Input: dimensioned drawing with shaded views. Units: mm. Origin: part minimum x, y, z. A direction names the side the tool comes from. Round coordinates to 2 decimals unless told otherwise and drop trailing zeros. Loops run counter-clockwise (first coordinate to the right, second up) from the corner with the lowest first, then second, coordinate; pieces in that order, holes last.
Item 1: Section query A-A on z = 16.5. Return loops of the section in (x, y), then the cut area to 3 significant figures.
Item 2: First-contact query: P1, Ø1.5, axis at y = 2.5, z = 10.5, coming from the +X side; P2, Ø2.5, axis at x = 6, z = 16.5, coming from the +Y side; P3, Ø0.9, axis at x = 6, z = 6.5, coming from the -Y side; P4, Ø2, axis at y = 3, z = 1, coming from the -X side. Flat tips, straight axial feed; report the tip coordinate or a pass-through.
Item 3: Section query B-B on y = 2.65. Return loops of the section in (x, z), then the cut area to 3 significant figures.
Item 4: Section query C-C on x = 2. Return loops of the section in (y, z), then the cut area to 3 significant figures.
Item 5: Section query D-D on x = 6. Return loops of the section in (y, z), then the cut area to 3 significant figures.
Item 6: Pull-direction query (Y, two-part tool) for the marked faces 4, 5 and 6; classes: released by +Y, released by -Y, zero draft, split by the parting line, or undercut.
Item 7: Ray query, L1, parallel to X at y = 2.25, z = 6; L2, parallel to X at y = 3.4, z = 16.5; L3, parallel to X at y = 1.05, z = 6.5. Return the intervals inside material, ascending.
Item 8: Access query for the marked faces 1, 2 and 3. Directions: +Z, -Z, +X, -X, +Y, -Y. A direction counts if a zero-diameter tool reaches every point of the face in a straight line with its end or side. Return the directions, or none.
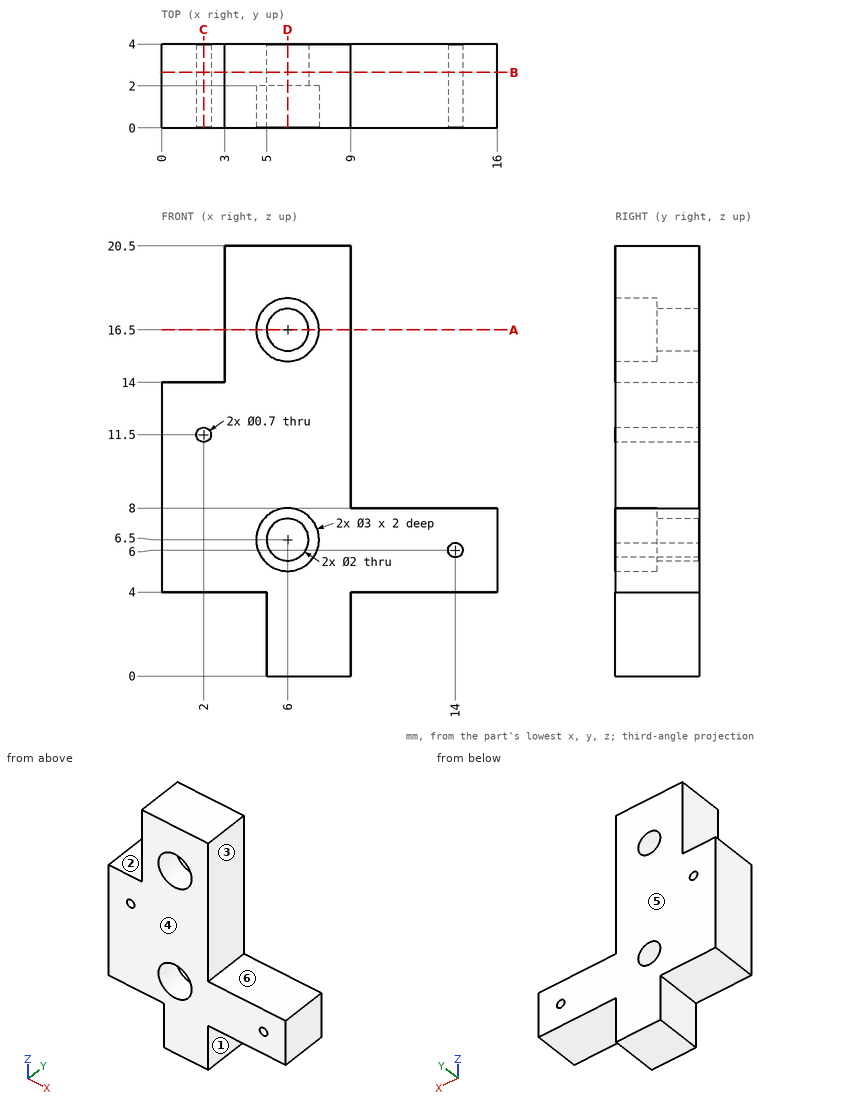
Data:
1. outline: (3, 0) - (4.5, 0) - (4.5, 2) - (5, 2) - (5, 4) - (3, 4) - close; (7, 2) - (7.5, 2) - (7.5, 0) - (9, 0) - (9, 4) - (7, 4) - close
1. area: 14.0 mm2
2. P1: stops at x = 9
2. P2: stops at y = 4
2. P3: passes through
2. P4: stops at x = 5
3. outline: (0, 4) - (5, 4) - (5, 0) - (9, 0) - (9, 4) - (16, 4) - (16, 8) - (9, 8) - (9, 20.5) - (3, 20.5) - (3, 14) - (0, 14) - close; hole circle Ø0.7 at (2, 11.5); hole circle Ø2 at (6, 6.5); hole circle Ø2 at (6, 16.5); hole circle Ø0.7 at (14, 6)
3. area: 166 mm2
4. outline: (0, 4) - (4, 4) - (4, 11.15) - (0, 11.15) - close; (0, 11.85) - (4, 11.85) - (4, 14) - (0, 14) - close
4. area: 37.2 mm2
5. outline: (0, 0) - (4, 0) - (4, 5.5) - (2, 5.5) - (2, 5) - (0, 5) - close; (0, 8) - (2, 8) - (2, 7.5) - (4, 7.5) - (4, 15.5) - (2, 15.5) - (2, 15) - (0, 15) - close; (0, 18) - (2, 18) - (2, 17.5) - (4, 17.5) - (4, 20.5) - (0, 20.5) - close
5. area: 62.0 mm2
6. face 4: released by -Y
6. face 5: released by +Y
6. face 6: zero draft
7. L1: x = 0 to 5.13, 6.87 to 13.65, 14.35 to 16
7. L2: x = 3 to 5, 7 to 9
7. L3: x = 0 to 4.5, 7.5 to 16
8. face 1: -Z, +X, +Y, -Y
8. face 2: +Z, -X, +Y, -Y
8. face 3: +Z, +X, +Y, -Y
